```python
from build123d import *

# Parameters (mm, degrees)
ESBO_O1_W                = 200
ESBO_O1_H                = 200
RESSALTO_EXTRUS_O1_DEPTH = 4
ESBO_O2_W                = 20
ESBO_O2_H                = 4
ESBO_O2_W_2              = 4
ESBO_O2_H_2              = 20
CORTE_EXTRUS_O1_DEPTH    = 5


with BuildPart() as part:
    # Esboço1 → Ressalto-extrusão1 (new body)
    with BuildSketch(Plane(origin=(0, 0, 0), x_dir=(1, 0, 0), z_dir=(0, 1, 0))):
        Rectangle(ESBO_O1_W, ESBO_O1_H)
    extrude(amount=RESSALTO_EXTRUS_O1_DEPTH)

    # Esboço2 → Corte-extrusão1 (cut, through all)
    with BuildSketch(Plane(origin=(0, 4, 0), x_dir=(1, 0, 0), z_dir=(0, 1, 0))):
        with Locations((-55, 98)):
            Rectangle(ESBO_O2_W, ESBO_O2_H)
        with Locations((55, 98)):
            Rectangle(ESBO_O2_W, ESBO_O2_H)
        with Locations((0, 98)):
            Rectangle(ESBO_O2_W, ESBO_O2_H)
        with Locations((98, 55)):
            Rectangle(ESBO_O2_W_2, ESBO_O2_H_2)
        with Locations((98, 0)):
            Rectangle(ESBO_O2_W_2, ESBO_O2_H_2)
        with Locations((98, -55)):
            Rectangle(ESBO_O2_W_2, ESBO_O2_H_2)
        with Locations((-98, 0)):
            Rectangle(ESBO_O2_W_2, ESBO_O2_H_2)
        with Locations((-98, -55)):
            Rectangle(ESBO_O2_W_2, ESBO_O2_H_2)
        with Locations((-98, 55)):
            Rectangle(ESBO_O2_W_2, ESBO_O2_H_2)
        with Locations((55, -98)):
            Rectangle(ESBO_O2_W, ESBO_O2_H)
        with Locations((-55, -98)):
            Rectangle(ESBO_O2_W, ESBO_O2_H)
        with Locations((0, -98)):
            Rectangle(ESBO_O2_W, ESBO_O2_H)
    extrude(amount=-CORTE_EXTRUS_O1_DEPTH, mode=Mode.SUBTRACT)


solid = part.part
```
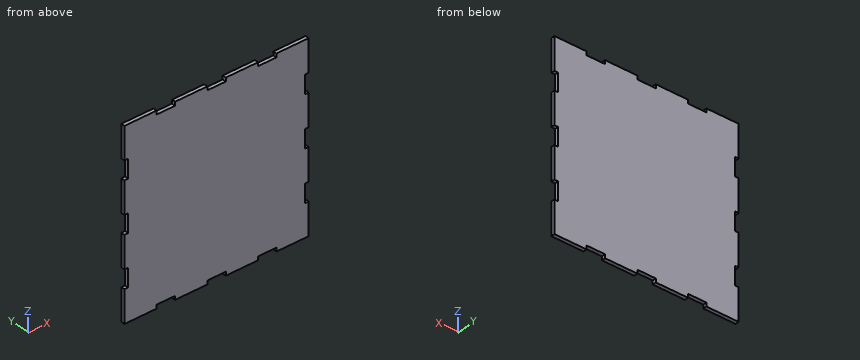
The listing builds one solid part. Answer for the finished solid, in the listing's coordinates (mm). Round coordinates to 2 decimals unless told otherwise and drop trailing zeros. Loops run counter-clockwise (first coordinate to the right, second up) from the corner with the lowest first, then second, coordinate; pieces in that order, holes last.
1) A cutting plane is placed at B-B on z = -49.5. Determine the outline of the cut face in (x, y).
Outcome:
outline: (-96, 0) - (96, 0) - (96, 4) - (-96, 4) - close
2) Given P1, Ø10, axis at x = -40.5, z = -54, coming from the -Y side; P2, Ø1, axis at x = -51, y = 2, coming from the -Z side, each flat-ended and moving along its own axis, determine where each tip first touches the part or whether it passes through.
Outcome:
P1: stops at y = 0
P2: stops at z = -96
3) A cutting plane is placed at A-A on x = -2. Determine the outline of the cut face in (y, z).
Outcome:
outline: (0, -96) - (4, -96) - (4, 96) - (0, 96) - close
4) Consider line 1 (X direction, y = 1.6, z = -52.5). Determine where the line is inside the solid, lowest interval first.
Outcome:
line 1: x = -96 to 96
